```python
from build123d import *

# Parameters (mm, degrees)
SKETCH2_R           = 5
BOSS_EXTRUDE1_DEPTH = 30
SKETCH1_R           = 9
BASE_EXTRUDE_DEPTH  = 4
CHAMFER1_SIZE       = 1
CHAMFER2_SIZE       = 2


with BuildPart() as part:
    # Sketch2 (on Front Plane) → Boss-Extrude1 (new body)
    with BuildSketch(Plane.XY):
        Circle(SKETCH2_R)
    extrude(amount=BOSS_EXTRUDE1_DEPTH)

    # Sketch1 → Base-Extrude (add)
    with BuildSketch(Plane.XY):
        Circle(SKETCH1_R)
    extrude(amount=-BASE_EXTRUDE_DEPTH)

    # Chamfer1
    chamfer1_edges = [part.edges().sort_by_distance(p)[0] for p in [
        (-9, 0, -4),
    ]]
    chamfer(chamfer1_edges, length=CHAMFER1_SIZE)

    # Chamfer2
    chamfer2_edges = [part.edges().sort_by_distance(p)[0] for p in [
        (-5, 0, 30),
    ]]
    chamfer(chamfer2_edges, length=CHAMFER2_SIZE)


solid = part.part
```
Can you work these out from the model? Positions are in its coordinate system, mm. A direction names the side the tool comes from. Round coordinates to 2 decimals unless told otherwise and drop trailing zeros. Loops run counter-clockwise (first coordinate to the right, second up) from the corner with the lowest first, then second, coordinate; pieces in that order, holes last. Notation, with made-up numbers: M -17.5,-31.5 L 29.5,-31.5 A36 ccw 29.5,4.5 Z; hole C -11.5,1 d6. An arc over 180 degrees is marked long. Write item = value, one per line. Start each with the question number.
(1) Which directions (+Z, -Z, +X, -X, +Y, -Y) give clear straight access to the entire face, cutting with the end or side of a thin tool? Please do faces 1 (the face through (0, 0, -4)), 2 (the face through (4, -4, 0)).
(2) Suppose I cut it at A-A on y = 0. Write out the boundary of the cut face in (x, z), plus the area to 3 significant figures.
(3) Suppose I cut it at C-C on z = 3. Write out the boundary of the cut face in (x, y), plus the area to 3 significant figures.
(4) I'm going to push flat-ended pins straight in: P1, Ø2, axis at y = -5.5, z = 3.5, coming from the +X side; P2, Ø8, axis at y = 7, z = 2.5, coming from the -X side; P3, Ø8, axis at y = -6.5, z = 13.5, coming from the -X side. Where does each tip first touch, or does it pass through?
(5) I need wall thicknesses on line 1 along X through (y, z) = (0.25, 6.5); line 2 along X through (y, z) = (-4, 11.5). Which ranges of each line are inside material? Lowest first, please.
(6) If we mould it in two halves opening along X, with no side actions, what happens to faces 3 (the face through (0, 0, 30)), 4 (the face through (-1.172, 8.923, -1.479))? For each: released by +X, released by -X, zero draft, split by the parting line, or undercut.
Answer block:
q1.face_1 = -Z, +X, -X, +Y, -Y
q1.face_2 = +Z
q2.outline = M -9,-3 L -8,-4 L 8,-4 L 9,-3 L 9,0 L 5,0 L 5,28 L 3,30 L -3,30 L -5,28 L -5,0 L -9,0 Z
q2.area = 367 mm²
q3.outline = C 0,0 d10
q3.area = 78.5 mm²
q4.P1 = 2.18
q4.P2 = -8.12
q4.P3 = -4.33
q5.line_1 = -4.99 to 4.99
q5.line_2 = -3 to 3
q6.face_3 = zero draft
q6.face_4 = split by the parting line
